```python
from build123d import *

# Parameters (mm, degrees)
SKETCH_1_W          = 39.6
SKETCH_1_H          = 70
EXTRUDE_1_DEPTH     = 3
HOLE_WIZARD_1_D     = 3.5
SKETCH_5_W          = 13
SKETCH_5_H          = 28
EXTRUDE_2_DEPTH     = 3
SKETCH_6_W          = 3
SKETCH_6_H          = 28
EXTRUDE_3_DEPTH     = 42
FILLET_1_R          = 10
FILLET_2_R          = 10
SKETCH_7_W          = 13
SKETCH_7_H          = 10.8
EXTRUDE_4_DEPTH     = 3
FILLET_4_R          = 3
SKETCH_8_W          = 15.6
SKETCH_8_H          = 15
CUT_EXTRUDE_1_DEPTH = 99.446736868
FILLET_5_R          = 5


with BuildPart() as part:
    # 草图1 → 凸台-拉伸1 (new body)
    with BuildSketch(Plane(origin=(0, 0, 0), x_dir=(1, 0, 0), z_dir=(0, 1, 0))):
        with Locations((19.8, 35)):
            Rectangle(SKETCH_1_W, SKETCH_1_H)
    extrude(amount=EXTRUDE_1_DEPTH)

    # 孔1 (through all)
    with Locations(Plane(origin=(0, 3, 0), x_dir=(1, 0, 0), z_dir=(0, 1, 0))):
        with Locations((6.8, 65), (32.8, 65)):
            Hole(HOLE_WIZARD_1_D / 2)

    # 草图5 → 凸台-拉伸2 (add)
    with BuildSketch(Plane(origin=(0, 3, 0), x_dir=(1, 0, 0), z_dir=(0, 1, 0))):
        with Locations((46.1, 36)):
            Rectangle(SKETCH_5_W, SKETCH_5_H)
        with Locations((-6.5, 36)):
            Rectangle(SKETCH_5_W, SKETCH_5_H)
    extrude(amount=-EXTRUDE_2_DEPTH)

    # 草图6 → 凸台-拉伸3 (add)
    with BuildSketch(Plane.XZ):
        with Locations((-11.5, -36)):
            Rectangle(SKETCH_6_W, SKETCH_6_H)
        with Locations((51.1, -36)):
            Rectangle(SKETCH_6_W, SKETCH_6_H)
    extrude(amount=EXTRUDE_3_DEPTH)

    # 圆角1
    fillet_1_edges = [part.edges().sort_by_distance(p)[0] for p in [
        (39.6, 1.5, -22),
        (0, 1.5, -22),
    ]]
    fillet(fillet_1_edges, radius=FILLET_1_R)

    # 圆角2
    fillet_2_edges = [part.edges().sort_by_distance(p)[0] for p in [
        (39.6, 1.5, 0),
        (0, 1.5, 0),
    ]]
    fillet(fillet_2_edges, radius=FILLET_2_R)

    # 草图7 → 凸台-拉伸4 (add)
    with BuildSketch(Plane(origin=(0, 3, 0), x_dir=(1, 0, 0), z_dir=(0, 1, 0))):
        with Locations((46.1, 55.4)):
            Rectangle(SKETCH_7_W, SKETCH_7_H)
        with Locations((-6.5, 55.4)):
            Rectangle(SKETCH_7_W, SKETCH_7_H)
    extrude(amount=-EXTRUDE_4_DEPTH)

    # 圆角4
    fillet_4_edges = [part.edges().sort_by_distance(p)[0] for p in [
        (52.6, 1.5, -60.8),
        (-13, 1.5, -60.8),
    ]]
    fillet(fillet_4_edges, radius=FILLET_4_R)

    # 草图8 → 切除-拉伸1 (cut, through all)
    with BuildSketch(Plane(origin=(0, 3, 0), x_dir=(1, 0, 0), z_dir=(0, 1, 0))):
        with Locations((19.8, 7.5)):
            Rectangle(SKETCH_8_W, SKETCH_8_H)
    extrude(amount=-CUT_EXTRUDE_1_DEPTH, mode=Mode.SUBTRACT)

    # 圆角5
    fillet_5_edges = [part.edges().sort_by_distance(p)[0] for p in [
        (12, 1.5, -15),
        (27.6, 1.5, -15),
    ]]
    fillet(fillet_5_edges, radius=FILLET_5_R)


solid = part.part
```
CAD build for the part. Positions are in the model's coordinates, mm. A direction names the side the tool comes from. Round coordinates to 2 decimals unless told otherwise and drop trailing zeros. Write each loop counter-clockwise with the first axis right and the second up, starting at its lowest first coordinate (ties: lowest second). Pieces come first, ordered by that corner, then holes. Notation, with made-up numbers: (21, -31) - (35, -31) arc R21 cw to (35, 7) - close; hole circle Ø7 at (49, -8.5). An arc over 180 degrees is marked (long way). Write item = value, one per line. Start each with the question number.
Q1. Probe L1, parallel to X at y = 1.3, z = -65; L2, parallel to X at y = -22, z = -44.5; L3, parallel to Y at x = 1, z = -60.5. List the from-to ranges inside material, lowest first. Write a range as from..to.
Q2. Mould opens along Z. For faces 1 (the flat face through (-5, 2, -60.8)), 2 (the cylindrical face through (7.18, 1.48, -63.29)), 3 (the flat face through (0, 1, -11)) say: pulls with the +Z half, pulls with the -Z half, needs draft (parallel to the pull), parting line crosses it, or undercut.
Q3. Band-saw the part on B-B (y = -21.5). Give the cut face in (x, z), then the cut area to 3 significant figures.
Q4. Band-saw the part on D-D (z = -32). Give the cut face in (x, y).
Q5. Which spindle directions (+Z, -Z, +X, -X, +Y, -Y) get a long thin tool onto all of the face, cutting with end or side? Do faces 4 (the flat face through (51, -21, -50)), 5 (the flat face through (20, 2, -15)), 6 (the flat face through (39.6, 1, -65)), 7 (the flat face through (49.6, -21, -36)), 8 (the flat face through (39.6, 1, -11)). Say none if no direction does.
Q6. Band-saw the part on A-A (z = -65). Give the cut face in (x, y).
Q7. Band-saw the part on C-C (x = 6.8). Give the cut face in (y, z), then the cut area to 3 significant figures.
Q8. Drop flat-ended pins along their axis: pin 1 (4 mm diameter, centred on x = 45, z = -49.5, fed in from -Y); pin 2 (2.5 mm diameter, centred on y = 1, z = -66, fed in from +X); pin 3 (0.9 mm diameter, centred on y = 1.5, z = -7, fed in from -X). Give the stop position or say it passes through.
Answers below:
q1.L1 = 0..5.05, 8.55..31.05, 34.55..39.6
q1.L2 = -13..-10, 49.6..52.6
q1.L3 = 0..3
q2.face_1 = pulls with the -Z half
q2.face_2 = undercut
q2.face_3 = needs draft
q3.outline = (-13, -50) - (-10, -50) - (-10, -22) - (-13, -22) - close; (49.6, -50) - (52.6, -50) - (52.6, -22) - (49.6, -22) - close
q3.area = 168 mm2
q4.outline = (-13, -42) - (-10, -42) - (-10, 0) - (49.6, 0) - (49.6, -42) - (52.6, -42) - (52.6, 3) - (-13, 3) - close
q5.face_4 = -Z, +X, -X, -Y
q5.face_5 = +Z, +Y, -Y
q5.face_6 = -Z, +X, +Y, -Y
q5.face_7 = +Z, -Z, -Y
q5.face_8 = +Z, +X, +Y, -Y
q6.outline = (0, 0) - (5.05, 0) - (5.05, 3) - (0, 3) - close; (8.55, 0) - (31.05, 0) - (31.05, 3) - (8.55, 3) - close; (34.55, 0) - (39.6, 0) - (39.6, 3) - (34.55, 3) - close
q7.outline = (0, -70) - (3, -70) - (3, -66.75) - (0, -66.75) - close; (0, -63.25) - (3, -63.25) - (3, -0.53) - (0, -0.53) - close
q7.area = 198 mm2
q8.pin_1 = 0
q8.pin_2 = 39.6
q8.pin_3 = 0.33
